For this review, take the finished solid that the model builds, in its own axes (mm). Round coordinates to 2 decimals unless told otherwise and drop trailing zeros. Order: outer loops, then holes, each group sorted by start corner. A loop starts at its lowest first (then second) coordinate and runs counter-clockwise, first axis right, second up. Notation, with made-up numbers: M -32.75,30 L -27.75,30 A32 cw -27.75,58 Z; hole C 37.25,45.5 d3. An arc over 180 degrees is marked long. Put each result on its own line as item: value.
from build123d import *

# Parameters (mm, degrees)
F1_DEPTH = 3


with BuildPart() as f1:
    # F0 (on Front) → F1 (new body)
    with BuildSketch(Plane.XZ):
        with BuildLine():
            Line((58.8, 11.4), (0, 11.4))
            ThreePointArc((0, 11.4), (-9.870808, 5.703258), (-9.87645, -5.693483))
            Line((-9.87645, -5.693483), (-0.07645, -22.693483))
            ThreePointArc((-0.07645, -22.693483), (4.096742, -26.870808), (9.8, -28.4))
            Line((9.8, -28.4), (68.6, -28.4))
            ThreePointArc((68.6, -28.4), (78.470808, -22.703258), (78.47645, -11.306517))
            Line((78.47645, -11.306517), (68.67645, 5.693483))
            ThreePointArc((68.67645, 5.693483), (64.503258, 9.870808), (58.8, 11.4))
        make_face()
        with BuildLine():
            ThreePointArc((-8.143739, -4.694626), (-8.139087, 4.702686), (0, 9.4))
            Line((0, 9.4), (19.6, 9.4))
            Line((19.6, 9.4), (39.2, 9.4))
            Line((39.2, 9.4), (58.8, 9.4))
            ThreePointArc((58.8, 9.4), (63.502686, 8.139087), (66.943739, 4.694626))
            Line((66.943739, 4.694626), (76.743739, -12.305374))
            ThreePointArc((76.743739, -12.305374), (77.680505, -14.570097), (78, -17))
            ThreePointArc((78, -17), (75.246804, -23.646804), (68.6, -26.4))
            Line((68.6, -26.4), (49, -26.4))
            Line((49, -26.4), (29.4, -26.4))
            Line((29.4, -26.4), (9.8, -26.4))
            ThreePointArc((9.8, -26.4), (5.097314, -25.139087), (1.656261, -21.694626))
            Line((1.656261, -21.694626), (-8.143739, -4.694626))
        make_face(mode=Mode.SUBTRACT)
        with BuildLine():
            ThreePointArc((0, 9.4), (6.646804, 6.646804), (9.4, 0))
            ThreePointArc((9.4, 0), (2.429903, -9.080505), (-8.143739, -4.694626))
            Line((-8.143739, -4.694626), (1.656261, -21.694626))
            ThreePointArc((1.656261, -21.694626), (7.370097, -7.919495), (19.2, -17))
            ThreePointArc((19.2, -17), (16.446804, -23.646804), (9.8, -26.4))
            Line((9.8, -26.4), (29.4, -26.4))
            Line((29.4, -26.4), (49, -26.4))
            Line((49, -26.4), (68.6, -26.4))
            ThreePointArc((68.6, -26.4), (60.460913, -12.297314), (76.743739, -12.305374))
            Line((76.743739, -12.305374), (66.943739, 4.694626))
            ThreePointArc((66.943739, 4.694626), (67.880505, 2.429903), (68.2, 0))
            ThreePointArc((68.2, 0), (52.153196, -6.646804), (58.8, 9.4))
            Line((58.8, 9.4), (39.2, 9.4))
            Line((39.2, 9.4), (19.6, 9.4))
            Line((19.6, 9.4), (0, 9.4))
        make_face()
        with BuildLine():
            ThreePointArc((38.8, -17), (36.046804, -23.646804), (29.4, -26.4))
            ThreePointArc((29.4, -26.4), (22.753196, -10.353196), (38.8, -17))
        make_face(mode=Mode.SUBTRACT)
        with BuildLine():
            ThreePointArc((58.4, -17), (55.646804, -23.646804), (49, -26.4))
            ThreePointArc((49, -26.4), (42.353196, -10.353196), (58.4, -17))
        make_face(mode=Mode.SUBTRACT)
        with BuildLine():
            ThreePointArc((29, 0), (12.953196, -6.646804), (19.6, 9.4))
            ThreePointArc((19.6, 9.4), (26.246804, 6.646804), (29, 0))
        make_face(mode=Mode.SUBTRACT)
        with BuildLine():
            ThreePointArc((48.6, 0), (32.553196, -6.646804), (39.2, 9.4))
            ThreePointArc((39.2, 9.4), (45.846804, 6.646804), (48.6, 0))
        make_face(mode=Mode.SUBTRACT)
    extrude(amount=F1_DEPTH)


solid = f1.part
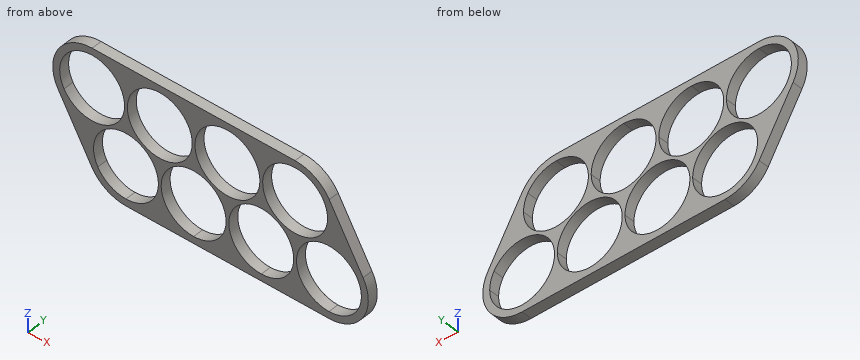
(1) To check wall thickness, follow L1, parallel to Z at x = 39.2, y = -1.8; L2, parallel to X at y = -2.15, z = -17; L3, parallel to X at y = -1.7, z = -4. State the ranges of each line that lie inside material, in increasing order.
A:
L1: z = -28.4 to -9.4, 9.4 to 11.4
L2: x = -3.36 to 0.4, 19.2 to 20, 38.8 to 39.6, 58.4 to 59.2, 78 to 80
L3: x = -10.68 to -8.51, 8.51 to 11.09, 28.11 to 30.69, 47.71 to 50.29, 67.31 to 74.26
(2) Add section D-D on x = 53. Give the boundary of the cut face in (y, z), then the cut area to 3 significant figures.
A:
outline: M -3,-28.4 L 0,-28.4 L 0,-25.51 L -3,-25.51 Z; M -3,-8.49 L 0,-8.49 L 0,-7.4 L -3,-7.4 Z; M -3,7.4 L 0,7.4 L 0,11.4 L -3,11.4 Z
area: 24.0 mm2
(3) Add section B-B on y = -0.8. State how many separate pieces and enclosed holes the cut face has, then the cut area to 3 significant figures.
A:
separate pieces: 1
enclosed holes: 8
area: 975 mm2
(4) Add section A-A on x = -3. Give the boundary of the cut face in (y, z), then the cut area to 3 significant figures.
A:
outline: M -3,-17.62 L 0,-17.62 L 0,-8.91 L -3,-8.91 Z; M -3,8.91 L 0,8.91 L 0,11 L -3,11 Z
area: 32.4 mm2
(5) Insertion check: pin 1 Ø17 at (x, z) = (19.6, 0) entering from +Y (3 decimals); pin 2 Ø1.5 at (y, z) = (-1, 3) entering from -X; pin 3 Ø5 at (x, z) = (44.5, -22.5) entering from +Y. Each pin has a flat end and moves straight along its axis. Give the tip position at first contact, or say it passes through.
A:
pin 1: passes through
pin 2: stops at x = -11.18
pin 3: stops at y = 0
(6) Add section C-C on z = 2. Give the boundary of the cut face in (x, y).
A:
outline: M -11.22,-3 L -9.18,-3 L -9.18,0 L -11.22,0 Z; M 9.18,-3 L 10.42,-3 L 10.42,0 L 9.18,0 Z; M 28.78,-3 L 30.02,-3 L 30.02,0 L 28.78,0 Z; M 48.38,-3 L 49.62,-3 L 49.62,0 L 48.38,0 Z; M 67.98,-3 L 70.81,-3 L 70.81,0 L 67.98,0 Z
